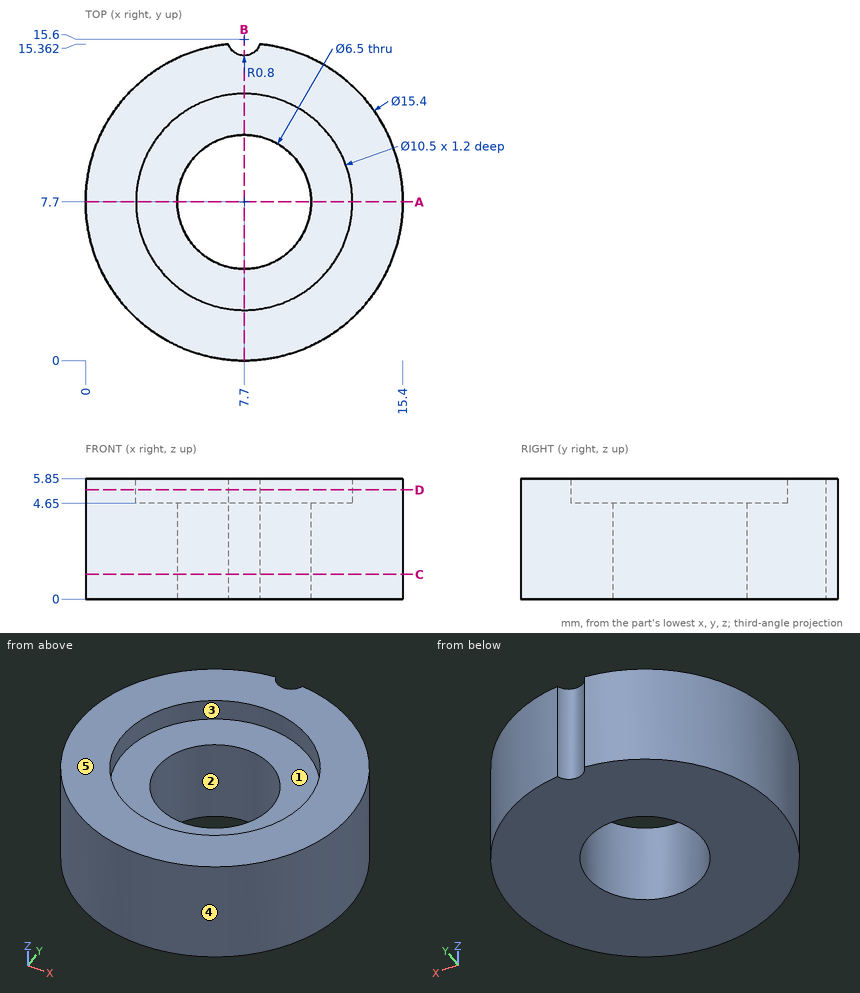
Part print with two shaded views. Sizes in mm from the minimum x, y, z corner. A direction names the side the tool comes from. Round coordinates to 2 decimals unless told otherwise and drop trailing zeros. Loops run counter-clockwise (first coordinate to the right, second up) from the corner with the lowest first, then second, coordinate; pieces in that order, holes last. Notation, with made-up numbers: (-24.75, -6.75) - (19.25, -6.75) arc R16 cw to (19.25, 21.25) - close; hole circle Ø11 at (-27.75, 22). An arc over 180 degrees is marked (long way). Put each result on its own line as item: value.
1. Slice it at A-A on y = 7.7. List the corners of the cut face in (x, z).
Geometry check:
outline: (0, 0) - (4.45, 0) - (4.45, 4.65) - (2.45, 4.65) - (2.45, 5.85) - (0, 5.85) - close; (10.95, 0) - (15.4, 0) - (15.4, 5.85) - (12.95, 5.85) - (12.95, 4.65) - (10.95, 4.65) - close
2. Slice it at D-D on z = 5.3. List the corners of the cut face in (x, y), and give its area (3 significant figures).
Geometry check:
outline: (6.94, 15.36) arc R7.7 ccw (long way) to (8.46, 15.36) arc R0.8 cw to start; hole circle Ø10.5 at (7.7, 7.7)
area: 99.0 mm²
3. Two-plate mould, pull along X, no slides. Class the marked faces 3, 4 and 5: released by +X, released by -X, zero draft, split by the parting line, or undercut.
Geometry check:
face 3: undercut
face 4: split by the parting line
face 5: zero draft
4. Wall check: line 1 (Y direction, x = 7.7, z = 5.5); line 2 (Y direction, x = 7.7, z = 1.65); line 3 (X direction, y = 8.75, z = 3.45). Give the ranges that are in metal, low to high.
Geometry check:
line 1: 0 to 2.45, 12.95 to 14.8
line 2: 0 to 4.45, 10.95 to 14.8
line 3: 0.07 to 4.62, 10.78 to 15.33
5. Pin check, flat tips, straight feed: P1, Ø3, axis at x = 10.5, z = 2.5, coming from the +Y side; P2, Ø1.5, axis at x = 10, z = 4.5, coming from the -Y side; P3, Ø3, axis at x = 7, y = 5, coming from the +Z side. Stop position of each tip, or through.
Geometry check:
P1: y = 15.29
P2: y = 0.16
P3: z = 4.65
6. Slice it at B-B on x = 7.7. List the corners of the cut face in (y, z), and give its area (3 significant figures).
Geometry check:
outline: (0, 0) - (4.45, 0) - (4.45, 4.65) - (2.45, 4.65) - (2.45, 5.85) - (0, 5.85) - close; (10.95, 0) - (14.8, 0) - (14.8, 5.85) - (12.95, 5.85) - (12.95, 4.65) - (10.95, 4.65) - close
area: 43.8 mm²
7. Slice it at C-C on z = 1.2. List the corners of the cut face in (x, y).
Geometry check:
outline: (6.94, 15.36) arc R7.7 ccw (long way) to (8.46, 15.36) arc R0.8 cw to start; hole circle Ø6.5 at (7.7, 7.7)
8. 3-axis set-ups, long thin cutter, end or side, ignore diameter. For the marked faces 1 and 2: which of +Z, -Z, +X, -X, +Y, -Y reach the whole face in a straight line?
Geometry check:
face 1: +Z
face 2: +Z, -Z
